Can you work these out from the model? Positions are in its coordinate system, mm. Give positions to 0.01 mm unless a question says otherwise; leave off trailing zeros. Order: outer loops, then holes, each group sorted by start corner. A loop starts at its lowest first (then second) coordinate and runs counter-clockwise, first axis right, second up. Notation, with made-up numbers: (75.25, 60) -> (95.25, 60) arc R22 cw to (95.25, 80) -> close; hole circle Ø1 at (-33, 24). An arc over 180 degrees is marked (long way). Answer as CSV lines item,"result".
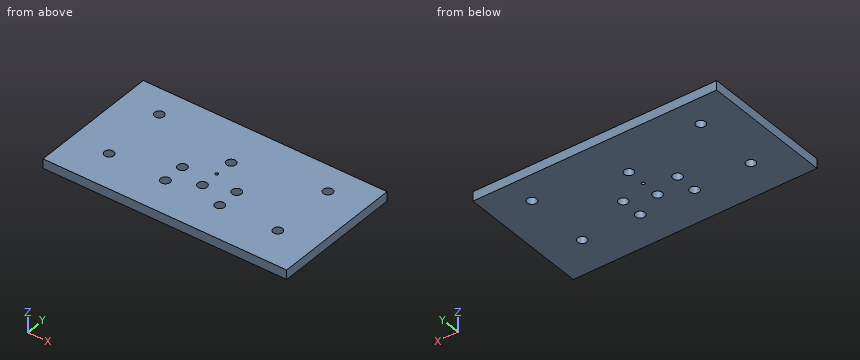
```python
from build123d import *

# Parameters (mm, degrees)
ESQUISSE1_W             = 130
ESQUISSE1_H             = 70
ESQUISSE1_R             = 2.5
BOSS_EXTRU_4_DEPTH      = 5
ESQUISSE2_R             = 0.8
ESQUISSE2_R_2           = 2.5
ENL_V_MAT_EXTRU_1_DEPTH = 10


with BuildPart() as part:
    # Esquisse1 → Boss.-Extru.4 (new body)
    with BuildSketch(Plane.XY):
        with Locations((65, 35)):
            Rectangle(ESQUISSE1_W, ESQUISSE1_H)
        with Locations((20, 55)):
            Circle(ESQUISSE1_R, mode=Mode.SUBTRACT)
        with Locations((110, 55)):
            Circle(ESQUISSE1_R, mode=Mode.SUBTRACT)
        with Locations((50.5, 31.23)):
            Circle(ESQUISSE1_R, mode=Mode.SUBTRACT)
        with Locations((79.5, 31.23)):
            Circle(ESQUISSE1_R, mode=Mode.SUBTRACT)
        with Locations((50.5, 19.37)):
            Circle(ESQUISSE1_R, mode=Mode.SUBTRACT)
        with Locations((79.5, 19.37)):
            Circle(ESQUISSE1_R, mode=Mode.SUBTRACT)
        with Locations((20, 20)):
            Circle(ESQUISSE1_R, mode=Mode.SUBTRACT)
        with Locations((110, 20)):
            Circle(ESQUISSE1_R, mode=Mode.SUBTRACT)
    extrude(amount=BOSS_EXTRU_4_DEPTH)

    # Esquisse2 → Enlèv. mat.-Extru.1 (cut)
    with BuildSketch(Plane.XY.offset(5)):
        with Locations((65, 36.23)):
            Circle(ESQUISSE2_R)
        with Locations((65, 26.23)):
            Circle(ESQUISSE2_R_2)
        with Locations((65, 46.23)):
            Circle(ESQUISSE2_R_2)
    extrude(amount=-ENL_V_MAT_EXTRU_1_DEPTH, mode=Mode.SUBTRACT)


solid = part.part
```
Item 1: Imagine slicing it at D-D, the plane y = 46.23. Please give me the cut outline in (x, z).
Numbers:
outline,"(0, 0) -> (62.5, 0) -> (62.5, 5) -> (0, 5) -> close; (67.5, 0) -> (130, 0) -> (130, 5) -> (67.5, 5) -> close"
Item 2: Imagine slicing it at B-B, the plane x = 110. Please give me the cut outline in (y, z).
Numbers:
outline,"(0, 0) -> (17.5, 0) -> (17.5, 5) -> (0, 5) -> close; (22.5, 0) -> (52.5, 0) -> (52.5, 5) -> (22.5, 5) -> close; (57.5, 0) -> (70, 0) -> (70, 5) -> (57.5, 5) -> close"
Item 3: Imagine slicing it at A-A, the plane y = 55. Please give me the cut outline in (x, z).
Numbers:
outline,"(0, 0) -> (17.5, 0) -> (17.5, 5) -> (0, 5) -> close; (22.5, 0) -> (107.5, 0) -> (107.5, 5) -> (22.5, 5) -> close; (112.5, 0) -> (130, 0) -> (130, 5) -> (112.5, 5) -> close"
Item 4: Imagine slicing it at C-C, the plane z = 2.6. Give the number of separate pieces and of enclosed holes in the cut face, then the cut area to 3 significant figures.
Numbers:
separate pieces,"1"
enclosed holes,"11"
area,"8,900 mm²"
Item 5: Please list where these lines run through material, in increasing order: line 1 along Y through (x, z) = (20, 2.1); line 2 along Y through (x, z) = (50.5, 2); line 3 along Y through (x, z) = (65, 2.15).
Numbers:
line 1,"y = 0 to 17.5, 22.5 to 52.5, 57.5 to 70"
line 2,"y = 0 to 16.87, 21.87 to 28.73, 33.73 to 70"
line 3,"y = 0 to 23.73, 28.73 to 35.43, 37.03 to 43.73, 48.73 to 70"
